Can you work these out from the drawing? Everything is in mm from the part's minimum corner. Coordinates: 2 decimals unless noted, no trailing zeros. Loops run counter-clockwise (first coordinate to the right, second up) from the corner with the lowest first, then second, coordinate; pieces in that order, holes last. Notation, with made-up numbers: (-15, 85) -> (29, 85) arc R13 ccw to (29, 96) -> close; hole circle Ø10 at (46, 68.25). An arc over 180 degrees is marked (long way). Put each result on its own line as item: value. Start each with the question number.
Item 1: Will these pins go through, and if not, where does the flat tip stop? P1, Ø2, axis at x = 65, y = 2, coming from the +Z side (1 decimal); P2, Ø12, axis at x = 211.32, z = 211.32, coming from the -Y side; P3, Ø4, axis at x = 158, y = 3.5, coming from the -Z side.
Item 2: If we section it at A-A on z = 130: Please give me the cut outline in (x, y).
Item 3: If we section it at D-D on z = 170.5: Please give me the cut outline in (x, y).
Item 4: If we section it at B-B on x = 97: Please give me the cut outline in (y, z).
Item 5: If we section it at C-C on y = 4: State how many separate pieces and enclosed holes the cut face has, plus the area to 3 significant figures.
Item 6: Please list where these lines run through material, in increasing order: L1, parallel to X at y = 5.75, z = 52 (1 decimal); L2, parallel to Z at x = 48.5, y = 7.5 (1 decimal); L3, parallel to Z at x = 234.5, y = 9.75. Write a range as from..to.
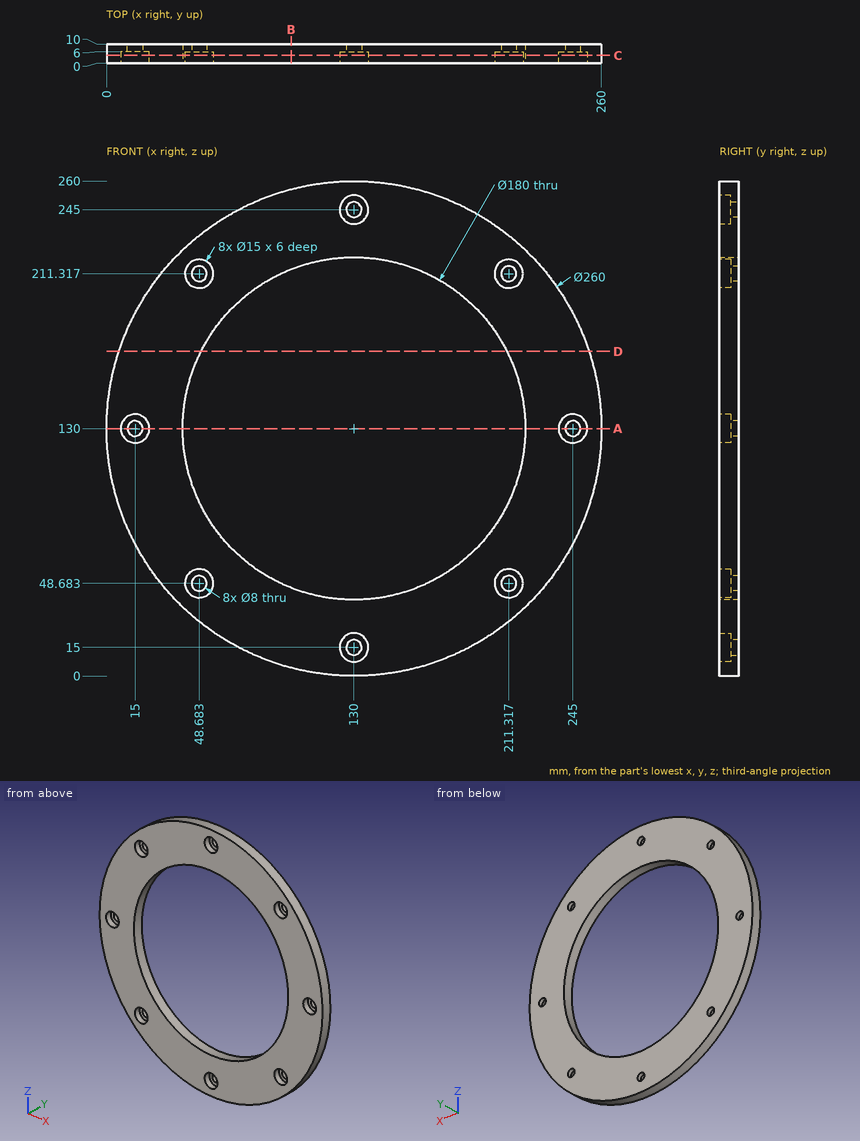
Solutions:
1. P1: z = 243.2
1. P2: y = 6
1. P3: z = 2.63
2. outline: (0, 0) -> (7.5, 0) -> (7.5, 6) -> (11, 6) -> (11, 10) -> (0, 10) -> close; (19, 6) -> (22.5, 6) -> (22.5, 0) -> (40, 0) -> (40, 10) -> (19, 10) -> close; (220, 0) -> (237.5, 0) -> (237.5, 6) -> (241, 6) -> (241, 10) -> (220, 10) -> close; (249, 6) -> (252.5, 6) -> (252.5, 0) -> (260, 0) -> (260, 10) -> (249, 10) -> close
3. outline: (6.47, 0) -> (49.63, 0) -> (49.63, 10) -> (6.47, 10) -> close; (210.37, 0) -> (253.53, 0) -> (253.53, 10) -> (210.37, 10) -> close
4. outline: (0, 4.26) -> (10, 4.26) -> (10, 46.27) -> (0, 46.27) -> close; (0, 213.73) -> (10, 213.73) -> (10, 255.74) -> (0, 255.74) -> close
5. separate pieces: 1
5. enclosed holes: 9
5. area: 26,200 mm^2
6. L1: 26..42, 55.4..85.1, 174.9..204.6, 218..234
6. L2: 28.7..44.7, 52.7..91.8, 168.2..207.3, 215.3..231.3
6. L3: 52.67..207.33
